Source: CAD feature listing. Evaluate the final solid. Frame: model axes, mm. A direction names the side the tool comes from. Round coordinates to 2 decimals unless told otherwise and drop trailing zeros. Write each loop counter-clockwise with the first axis right and the second up, starting at its lowest first coordinate (ties: lowest second). Pieces come first, ordered by that corner, then holes. Notation, with made-up numbers: M 19,25.25 L 56,25.25 A10 cw 56,39.25 Z; hole C 89.25,36.5 d6. An arc over 180 degrees is marked long. Put each result on its own line as item: value. Start each with the question number.
```python
from build123d import *

# Parameters (mm, degrees)
SKETCH_1_W          = 100
SKETCH_1_H          = 120
SKETCH_1_R          = 4
EXTRUDE_1_DEPTH     = 20
SKETCH_4_W          = 100
SKETCH_4_H          = 40
EXTRUDE_2_DEPTH     = 20
SKETCH_5_W          = 30
SKETCH_5_H          = 30
CUT_EXTRUDE_1_DEPTH = 10
SKETCH_7_R          = 5
CUT_EXTRUDE_3_DEPTH = 110
SKETCH_8_R          = 5
CUT_EXTRUDE_4_DEPTH = 1
SKETCH_9_W          = 20
SKETCH_9_H          = 100
CUT_EXTRUDE_6_DEPTH = 99.994949366
FILLET_5_R          = 10
FILLET_2_R          = 10
FILLET_1_R          = 10
FILLET_9_R          = 10


with BuildPart() as part:
    # ｽｹｯﾁ1 → ﾎﾞｽ - 押し出し1 (new body)
    with BuildSketch(Plane(origin=(0, 0, 0), x_dir=(1, 0, 0), z_dir=(0, 1, 0))):
        Rectangle(SKETCH_1_W, SKETCH_1_H)
        with Locations(Location((-20, -40, 0), (0, 0, 270))):
            Circle(SKETCH_1_R, mode=Mode.SUBTRACT)
        with Locations(Location((20, -40, 0), (0, 0, 270))):
            Circle(SKETCH_1_R, mode=Mode.SUBTRACT)
    extrude(amount=EXTRUDE_1_DEPTH)

    # ｽｹｯﾁ4 → ﾎﾞｽ - 押し出し2 (add)
    with BuildSketch(Plane.XY.offset(60)):
        with Locations((0, 10)):
            Rectangle(SKETCH_4_W, SKETCH_4_H)
    extrude(amount=EXTRUDE_2_DEPTH)

    # ｽｹｯﾁ5 → ｶｯﾄ - 押し出し1 (cut)
    with BuildSketch(Plane.XY.offset(80)):
        with Locations((0, 10)):
            Rectangle(SKETCH_5_W, SKETCH_5_H)
    extrude(amount=-CUT_EXTRUDE_1_DEPTH, mode=Mode.SUBTRACT)

    # ｽｹｯﾁ7 → ｶｯﾄ - 押し出し3 (cut)
    with BuildSketch(Plane.XY.offset(70)):
        with Locations((0, 10)):
            Circle(SKETCH_7_R)
    extrude(amount=-CUT_EXTRUDE_3_DEPTH, mode=Mode.SUBTRACT)

    # ｽｹｯﾁ8 → ｶｯﾄ - 押し出し4 (cut)
    with BuildSketch(Plane.XY.offset(80)):
        with Locations((-40, 20)):
            Circle(SKETCH_8_R)
        with Locations(Location((40, 20, 0), (0, 0, 180))):
            Circle(SKETCH_8_R)
        with Locations((40, 0)):
            Circle(SKETCH_8_R)
        with Locations(Location((-40, 0, 0), (0, 0, 180))):
            Circle(SKETCH_8_R)
    extrude(amount=-CUT_EXTRUDE_4_DEPTH, mode=Mode.SUBTRACT)

    # ｽｹｯﾁ9 → ｶｯﾄ - 押し出し6 (cut, through all)
    with BuildSketch(Plane(origin=(0, 20, 0), x_dir=(1, 0, 0), z_dir=(0, 1, 0))):
        with Locations((0, -10)):
            Rectangle(SKETCH_9_W, SKETCH_9_H)
    extrude(amount=-CUT_EXTRUDE_6_DEPTH, mode=Mode.SUBTRACT)

    # ﾌｨﾚｯﾄ5
    fillet_5_edges = [part.edges().sort_by_distance(p)[0] for p in [
        (15, 25, 75),
        (15, -5, 75),
        (-15, -5, 75),
        (-15, 25, 75),
    ]]
    fillet(fillet_5_edges, radius=FILLET_5_R)

    # ﾌｨﾚｯﾄ2
    fillet_2_edges = [part.edges().sort_by_distance(p)[0] for p in [
        (-50, 10, -60),
        (50, 10, -60),
    ]]
    fillet(fillet_2_edges, radius=FILLET_2_R)

    # ﾌｨﾚｯﾄ1
    fillet_1_edges = [part.edges().sort_by_distance(p)[0] for p in [
        (50, 30, 70),
        (50, -10, 70),
        (-50, -10, 70),
        (-50, 30, 70),
    ]]
    fillet(fillet_1_edges, radius=FILLET_1_R)

    # ﾌｨﾚｯﾄ9
    fillet_9_edges = [part.edges().sort_by_distance(p)[0] for p in [
        (-10, 10, -40),
        (10, 10, -40),
    ]]
    fillet(fillet_9_edges, radius=FILLET_9_R - 0.0001)  # a hair under: the kernel refuses the full size


solid = part.part
```
(1) Section query A-A (z = 40). Return loops of the section in (x, y), and give its area (3 significant figures).
(2) Pull-direction query (Y, two-part tool) for faces 1 (the flat face through (-40, 0, 79)), 2 (the flat face through (-12, 24, 80)), 3 (the flat face through (40, 20, 79)), 4 (the flat face through (-12, 0, -1)); classes: +Y half, -Y half, draft (parallel to the pull), parting line (faces both ways), or undercut.
(3) Section query B-B (z = 15). Return loops of the section in (x, y).
(4) Section query D-D (y = 13). Count the separate pieces of the cut face and the enclosed holes in it, and give its area (3 significant figures).
(5) Section query C-C (x = 33.5). Return loops of the section in (y, z).
(6) Contact query for flat-ended pins moving along their axis: P1, Ø3, axis at x = 10, y = 7, coming from the +Z side; P2, Ø1.5, axis at x = 8, z = 23.5, coming from the +Y side; P3, Ø6, axis at x = -40, y = 0, coming from the +Z side; P4, Ø6, axis at x = 11, z = 42.5, coming from the -Y side. Output: stop coordinate, or through.
(7) Access query for faces 5 (the flat face through (-12, 20, -1)), 6 (the flat face through (-10, 10, 16)), 7 (the cylindrical face through (46.99, -7.15, 70.14)), 8 (the flat face through (-4, 14, 70)). Directions: +Z, -Z, +X, -X, +Y, -Y. A direction counts if a zero-diameter tool reaches every point of the face in a straight line with its end or side. Return the directions, or none.
(8) Ray query, line 1 along X through (y, z) = (15.5, 40); line 2 along Y through (x, z) = (40, 79.6); line 3 along X through (y, z) = (14, -20). Return the intervals inside material, ascending.
Entries:
1. outline: M -50,0 L -24,0 L -24,20 L -50,20 Z; M -16,0 L -10,0 L -10,20 L -16,20 Z; M 10,0 L 16,0 L 16,20 L 10,20 Z; M 24,0 L 50,0 L 50,20 L 24,20 Z
1. area: 1,280 mm2
2. face 1: undercut
2. face 2: draft
2. face 3: undercut
2. face 4: -Y half
3. outline: M -50,0 L -10,0 L -10,20 L -50,20 Z; M 10,0 L 50,0 L 50,20 L 10,20 Z
4. separate pieces: 1
4. enclosed holes: 2
4. area: 11,500 mm2
5. outline: M -10,60 L 0,60 L 0,-60 L 20,-60 L 20,60 L 30,60 L 30,80 L -10,80 Z
6. P1: z = 70
6. P2: through
6. P3: z = 79
6. P4: y = 0
7. face 5: -Z, +X, -X, +Y
7. face 6: +Y, -Y
7. face 7: +Z, -Z, +X, -Y
7. face 8: +Z
8. line 1: -50 to -24, -16 to -10, 10 to 16, 24 to 50
8. line 2: -10 to -5, 5 to 15, 25 to 30
8. line 3: -50 to -10, 10 to 50
